The model under review builds one solid part; all positions refer to its coordinate system, in mm. Round coordinates to 2 decimals unless told otherwise and drop trailing zeros. Order: outer loops, then holes, each group sorted by start corner. A loop starts at its lowest first (then second) coordinate and runs counter-clockwise, first axis right, second up.
1) To check wall thickness, follow L1, parallel to Z at x = 8, y = 3.75; L2, parallel to Y at x = 7.25, z = 4.5; L3, parallel to X at y = 9.75, z = 4.25. State the ranges of each line that lie inside material, in increasing order.
2) Consider section A-A (y = 4). Give the boundary of the cut face in (x, z), then the cut area to 3 significant figures.
3) Clearance check with flat-ended pins moving along their axes: P1, Ø1.5, axis at x = 2, z = 7, coming from the -Y side; P2, Ø1.5, axis at y = 6.5, z = 6, coming from the +X side. State where each tip first meets the part, or that it passes through.
from build123d import *

# Parameters (mm, degrees)
F0_W     = 10.16
F0_H     = 10.16
F1_DEPTH = 8.89
F2_SIZE2 = 5.08
F2_SIZE  = 1.27
F3_R     = 2.54
F4_R     = 1.27


with BuildPart() as f1:
    # F0 (on Top) → F1 (new body)
    with BuildSketch(Plane.XY):
        with Locations((5.08, 5.08)):
            Rectangle(F0_W, F0_H)
    extrude(amount=F1_DEPTH)

    # F2
    f2_edges = [f1.edges().sort_by_distance(p)[0] for p in [
        (10.16, 5.08, 8.89),
        (5.08, 0, 8.89),
        (0, 5.08, 8.89),
        (5.08, 10.16, 8.89),
    ]]
    f2_side = f1.faces().sort_by_distance((5.08, 5.08, 8.89))[0]
    chamfer(f2_edges, length=F2_SIZE, length2=F2_SIZE2, reference=f2_side)

    # F3
    f3_edges = [f1.edges().sort_by_distance(p)[0] for p in [
        (9.525, 0.635, 6.35),
        (9.525, 9.525, 6.35),
        (0.635, 9.525, 6.35),
        (0.635, 0.635, 6.35),
    ]]
    fillet(f3_edges, radius=F3_R)

    # F4
    f4_edges = [f1.edges().sort_by_distance(p)[0] for p in [
        (1.983172, 8.176828, 8.89),
    ]]
    fillet(f4_edges, radius=F4_R)


solid = f1.part
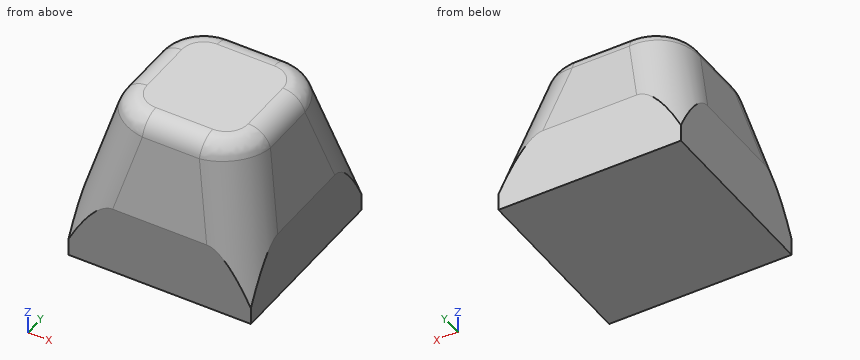
Answer below:
1. L1: z = 0 to 8.89
1. L2: y = 0.17 to 9.99
1. L3: x = 1.38 to 8.78
2. outline: (0, 0) - (10.16, 0) - (10.16, 3.81) - (9.13, 7.93) arc R1.27 ccw to (7.9, 8.89) - (2.26, 8.89) arc R1.27 ccw to (1.03, 7.93) - (0, 3.81) - close
2. area: 83.5 mm2
3. P1: stops at y = 0.73
3. P2: stops at x = 9.8
